```python
from build123d import *

# Parameters (mm, degrees)
SKETCH1_R                       = 3.175
BOSS_EXTRUDE1_DEPTH             = 241.3
F_6_32_TAPPED_HOLE1_D           = 2.7051
F_6_32_TAPPED_HOLE1_DEPTH       = 9.398
F_6_32_TAPPED_HOLE1_CBORE_D     = 3.5052
F_6_32_TAPPED_HOLE1_CBORE_DEPTH = 7.112
F_6_32_TAPPED_HOLE1_TIP         = 0.81269403
F_6_32_TAPPED_HOLE2_D           = 2.7051
F_6_32_TAPPED_HOLE2_DEPTH       = 9.398
F_6_32_TAPPED_HOLE2_CBORE_D     = 3.5052
F_6_32_TAPPED_HOLE2_CBORE_DEPTH = 7.112
F_6_32_TAPPED_HOLE2_TIP         = 0.81269403


with BuildPart() as part:
    # Sketch1 → Boss-Extrude1 (new body)
    with BuildSketch(Plane.XY):
        Circle(SKETCH1_R)
    extrude(amount=BOSS_EXTRUDE1_DEPTH)

    # #6-32 Tapped Hole1
    with Locations(Plane.XY.offset(241.3)):
        with Locations((0, 0)):
            CounterBoreHole(F_6_32_TAPPED_HOLE1_D / 2, F_6_32_TAPPED_HOLE1_CBORE_D / 2, F_6_32_TAPPED_HOLE1_CBORE_DEPTH, depth=F_6_32_TAPPED_HOLE1_DEPTH)
            with Locations((0, 0, -(F_6_32_TAPPED_HOLE1_DEPTH + F_6_32_TAPPED_HOLE1_TIP / 2))):  # 118° drill point
                Cone(0, F_6_32_TAPPED_HOLE1_D / 2, F_6_32_TAPPED_HOLE1_TIP, mode=Mode.SUBTRACT)

    # #6-32 Tapped Hole2
    with Locations(Plane(origin=(0, 0, 0), x_dir=(-1, 0, 0), z_dir=(0, 0, -1))):
        with Locations((0, 0)):
            CounterBoreHole(F_6_32_TAPPED_HOLE2_D / 2, F_6_32_TAPPED_HOLE2_CBORE_D / 2, F_6_32_TAPPED_HOLE2_CBORE_DEPTH, depth=F_6_32_TAPPED_HOLE2_DEPTH)
            with Locations((0, 0, -(F_6_32_TAPPED_HOLE2_DEPTH + F_6_32_TAPPED_HOLE2_TIP / 2))):  # 118° drill point
                Cone(0, F_6_32_TAPPED_HOLE2_D / 2, F_6_32_TAPPED_HOLE2_TIP, mode=Mode.SUBTRACT)


solid = part.part
```
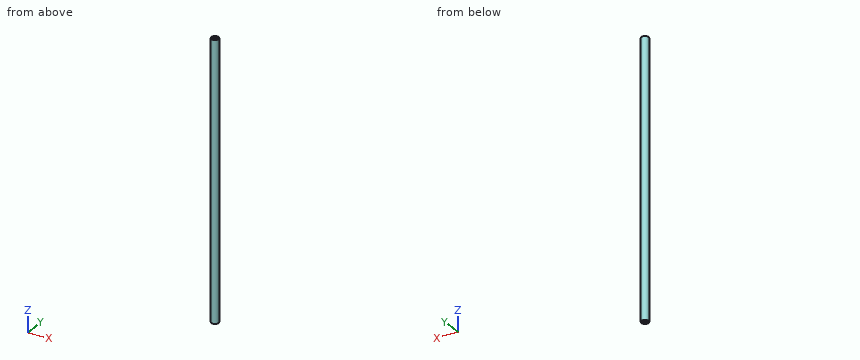
The model under review builds one solid part; all positions refer to its coordinate system, in mm. Round coordinates to 2 decimals unless told otherwise and drop trailing zeros. Loops run counter-clockwise (first coordinate to the right, second up) from the corner with the lowest first, then second, coordinate; pieces in that order, holes last. Notation, with made-up numbers: (16, 38) - (48, 38) arc R20 cw to (48, 55) - close; hole circle Ø7 at (23.5, -37). An arc over 180 degrees is marked (long way). Use a Markdown table: item, result. Add a question column.
Q1. Insertion check: pin 1 Ø2 at (x, y) = (0, 0) entering from -Z; pin 2 Ø2 at (x, y) = (0, 0) entering from +Z; pin 3 Ø1.8 at (x, y) = (0, 0) entering from +Z. Each pin has a flat end and moves straight along its axis. Give the tip position at first contact, or say it passes through.
Q2. For probe 1 along Y at (x, z) = (0, 2) (3 decimals); probe 2 along Z at (x, y) = (0.5, 1.5); probe 3 along Y at (x, z) = (0, 233.2) (3 decimals), list the stretches that pass through material, from the lowest coordinate up.
Q3. Add section A-A (z = 149.5). State the section outline as (x, y) points (3 decimals).
Worked answers:
| question | item | result |
|---|---|---|
| 1 | pin 1 | z = 9.61 |
| 1 | pin 2 | z = 231.69 |
| 1 | pin 3 | z = 231.63 |
| 2 | probe 1 | -3.175 to -1.753, 1.753 to 3.175 |
| 2 | probe 2 | 7.11 to 234.19 |
| 2 | probe 3 | -3.175 to -1.353, 1.353 to 3.175 |
| 3 | outline | circle Ø6.35 at (0, 0) |
